from build123d import *

# Parameters (mm, degrees)
MODEL_R         = 1.5999968
MODEL_R_2       = 2.0999958
MODEL_R_3       = 11.499977
EXTRUDE_1_DEPTH = 4


with BuildPart() as part:
    # Model → Бобышка-Вытянуть1 (new body)
    with BuildSketch(Plane.XY):
        with BuildLine():
            Line((274.028195208, 189.164211852), (274.028195208, 151.235355522))
            ThreePointArc((274.028195208, 151.235355522), (273.647593631, 149.321942187), (272.563732042, 147.699828687))
            Line((272.563732042, 147.699828687), (265.492678373, 140.628775017))
            ThreePointArc((265.492678373, 140.628775017), (264.408816784, 139.006661518), (264.028215208, 137.093248183))
            Line((264.028215208, 137.093248183), (264.028215208, 124.164341852))
            ThreePointArc((264.028215208, 124.164341852), (262.563752042, 120.628815017), (259.028225208, 119.164351852))
            Line((259.028225208, 119.164351852), (249.028245208, 119.164351852))
            ThreePointArc((249.028245208, 119.164351852), (245.492718373, 117.699888687), (244.028255208, 114.164361852))
            Line((244.028255208, 114.164361852), (244.028255208, 104.164381852))
            ThreePointArc((244.028255208, 104.164381852), (242.563792042, 100.628855017), (239.028265208, 99.164391852))
            Line((239.028265208, 99.164391852), (229.028285208, 99.164391852))
            ThreePointArc((229.028285208, 99.164391852), (225.492758373, 100.628855017), (224.028295208, 104.164381852))
            Line((224.028295208, 104.164381852), (224.028295208, 189.164211852))
            ThreePointArc((224.028295208, 189.164211852), (225.492758373, 192.699738687), (229.028285208, 194.164201852))
            Line((229.028285208, 194.164201852), (269.028205208, 194.164201852))
            ThreePointArc((269.028205208, 194.164201852), (272.563732043, 192.699738687), (274.028195208, 189.164211852))
        make_face()
        with Locations((267.528208208, 184.664220852)):
            Circle(MODEL_R, mode=Mode.SUBTRACT)
        with Locations((267.528208208, 153.664282852)):
            Circle(MODEL_R, mode=Mode.SUBTRACT)
        with Locations((236.528270208, 153.664282852)):
            Circle(MODEL_R, mode=Mode.SUBTRACT)
        with Locations((236.528270208, 184.664220852)):
            Circle(MODEL_R, mode=Mode.SUBTRACT)
        with Locations((254.028235208, 127.164335852)):
            Circle(MODEL_R_2, mode=Mode.SUBTRACT)
        with Locations((234.028275208, 127.164335852)):
            Circle(MODEL_R_2, mode=Mode.SUBTRACT)
        with Locations((234.028275208, 109.164371852)):
            Circle(MODEL_R_2, mode=Mode.SUBTRACT)
        with Locations((252.028239208, 169.164251852)):
            Circle(MODEL_R_3, mode=Mode.SUBTRACT)
    extrude(amount=EXTRUDE_1_DEPTH)


solid = part.part
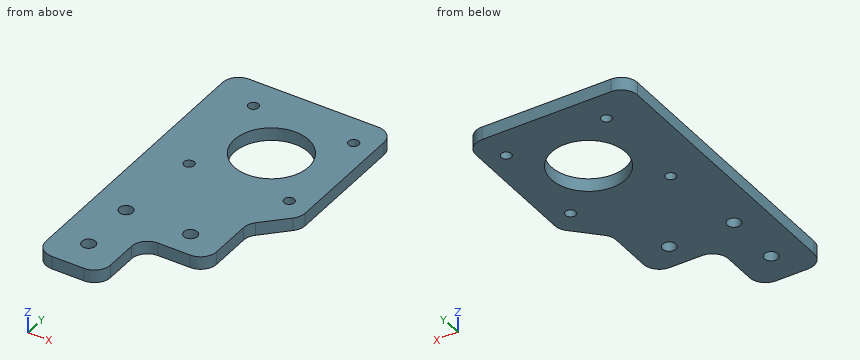
The model under review builds one solid part; all positions refer to its coordinate system, in mm. Round coordinates to 2 decimals unless told otherwise and drop trailing zeros. Loops run counter-clockwise (first coordinate to the right, second up) from the corner with the lowest first, then second, coordinate; pieces in that order, holes last. Notation, with made-up numbers: (26, 24) -> (38, 24) arc R22 ccw to (38, 52) -> close; hole circle Ø10 at (40.5, 49.25). An arc over 180 degrees is marked (long way). Return JSON: item names as keys, results as strings.
(1) Add section C-C on x = 262. Write out the cut boundary in (y, z).
Solved:
{"outline": "(120.14, 0) -> (163.44, 0) -> (163.44, 4) -> (120.14, 4) -> close; (174.89, 0) -> (194.16, 0) -> (194.16, 4) -> (174.89, 4) -> close"}
(2) Add section D-D on y = 112.5. Write out the cut boundary in (x, z), plus the area to 3 significant figures.
Solved:
{"outline": "(224.03, 0) -> (244.03, 0) -> (244.03, 4) -> (224.03, 4) -> close", "area": "80.0 mm2"}
(3) For pin 1 (2.5 mm diameter, centred on x = 236.53, y = 184.66, fed in from -Z); pin 2 (2 mm diameter, centred on x = 256, z = 2, fed in from -Y); pin 3 (1.2 mm diameter, centred on y = 108, z = 1.5, fed in from +X); pin 4 (2 mm diameter, centred on y = 131, z = 3, fed in from +X), all flat-tipped, find the tip position at first contact; note any pin that passes through.
Solved:
{"pin 1": "through", "pin 2": "y = 119.16", "pin 3": "x = 244.03", "pin 4": "x = 264.03"}
(4) Add section A-A on z = 0.7. State how many separate pieces and enclosed holes the cut face has, plus the area to 3 significant figures.
Solved:
{"separate pieces": "1", "enclosed holes": "8", "area": "3,390 mm2"}
(5) For line 1 (Y direction, x = 234, z = 2.6); line 2 (X direction, y = 177, z = 0.4); line 3 (X direction, y = 163.5, z = 3.25), list the stretches that pass through material, from the lowest coordinate up.
Solved:
{"line 1": "99.16 to 107.06, 111.26 to 125.06, 129.26 to 194.16", "line 2": "224.03 to 243.61, 260.45 to 274.03", "line 3": "224.03 to 242.02, 262.04 to 274.03"}
(6) Add section B-B on y = 171. Write out the cut boundary in (x, z).
Solved:
{"outline": "(224.03, 0) -> (240.68, 0) -> (240.68, 4) -> (224.03, 4) -> close; (263.38, 0) -> (274.03, 0) -> (274.03, 4) -> (263.38, 4) -> close"}
